Verification items for the finished model (mm, model axes). A direction names the side the tool comes from. Give positions to 0.01 mm unless a question says otherwise; leave off trailing zeros. Order: outer loops, then holes, each group sorted by start corner. A loop starts at its lowest first (then second) coordinate and runs counter-clockwise, first axis right, second up. Notation, with made-up numbers: (52, 66) -> (88, 66) arc R31 cw to (88, 93) -> close; hole circle Ø3 at (35, 33). An arc over 180 degrees is marked (long way). Return JSON: item names as keys, results as strings. Group by question number.
(1) Thickness scan on line 1 along X through (y, z) = (9.5, -14); line 2 along X through (y, z) = (2, -7); line 3 along Y through (x, z) = (20.5, 17.5). Record the ranges inside material, lowest first.
(2) Cross-section at D-D on x = 0. Enter the section's corners in (y, z), then the cut area to 3 significant figures.
(3) Tool access check on faces 4 (the face through (-22.43, 1.48, 23.27)), 5 (the face through (-28, 5, 5)), 6 (the face through (26, 5, -10)), 7 (the face through (24, 7, -10)). Record the directions out of +Z, -Z, +X, -X, +Y, -Y that give a thin tool (end or side, any length) a straight path to the whole face; none if there is none.
(4) Cross-section at C-C on z = -23. Enter the section's corners in (x, y).
(5) Release check for a two-part mould opening along X. For faces 1 (the face through (20, 1, 24.662)), 2 (the face through (-26, 5, -27)), 3 (the face through (28, 5, 5)) record: pulls with the +X half, pulls with the -X half, needs draft (parallel to the pull), parting line crosses it, or undercut.
(6) Depth check by flat-ended pin: pin 1 Ø5 at (x, y) = (-17, 4.5) entering from -Z; pin 2 Ø1.6 at (x, y) = (24.5, 7) entering from +Z; pin 3 Ø1 at (y, z) = (6.5, -8) entering from -X; pin 4 Ø4.5 at (x, z) = (0, 14) entering from -Y. Enter the tip coordinate at first touch or a pass-through.
(7) Cross-section at A-A on y = 6. Enter the section's corners in (x, z).
(8) Cross-section at B-B on x = -8. Enter the section's corners in (y, z).
from build123d import *

# Parameters (mm, degrees)
SKETCH1_W               = 52
SKETCH1_H               = 60
BOSS_EXTRUDE1_DEPTH     = 10
CUT_EXTRUDE1_DEPTH      = 5
SKETCH3_R               = 1.25
CUT_EXTRUDE2_DEPTH      = 5
CUT_EXTRUDE3_DEPTH      = 3
SKETCH6_W               = 24
SKETCH6_H               = 30
CUT_EXTRUDE4_DEPTH      = 41.938978981
SKETCH7_W               = 3
SKETCH7_H               = 10
BOSS_EXTRUDE2_DEPTH     = 10
LPATTERN1_COUNT         = 2
LPATTERN1_PITCH         = 20
MIRROR1_COPY_1_SKETCH_W = 3
MIRROR1_COPY_1_SKETCH_H = 10
MIRROR1_COPY_1_DEPTH    = 10
SKETCH8_W               = 48
SKETCH8_H               = 40
CUT_EXTRUDE5_DEPTH      = 2


with BuildPart() as part:
    # Sketch1 → Boss-Extrude1 (new body)
    with BuildSketch(Plane(origin=(0, 0, 0), x_dir=(1, 0, 0), z_dir=(0, 1, 0))):
        Rectangle(SKETCH1_W, SKETCH1_H)
    extrude(amount=BOSS_EXTRUDE1_DEPTH)

    # Sketch2 → Cut-Extrude1 (cut)
    with BuildSketch(Plane(origin=(0, 10, 0), x_dir=(1, 0, 0), z_dir=(0, 1, 0))):
        Polygon((-26, -30), (26, -30), (26, -10), (24, -10), (24, 30), (-24, 30), (-24, -10), (-26, -10), align=None)
    extrude(amount=-CUT_EXTRUDE1_DEPTH, mode=Mode.SUBTRACT)

    # Sketch3 → Cut-Extrude2 (cut)
    with BuildSketch(Plane(origin=(0, 5, 0), x_dir=(1, 0, 0), z_dir=(0, 1, 0))):
        with Locations(Location((-20, -21.847557332, 0), (0, 0, 270))):
            Circle(SKETCH3_R)
        with Locations(Location((0, -13.847557332, 0), (0, 0, 270))):
            Circle(SKETCH3_R)
        with Locations(Location((20, -21.847557332, 0), (0, 0, 270))):
            Circle(SKETCH3_R)
    extrude(amount=-CUT_EXTRUDE2_DEPTH, mode=Mode.SUBTRACT)

    # Sketch5 → Cut-Extrude3 (cut)
    with BuildSketch(Plane.XZ):
        Polygon((-18.375, 24.662139894), (-21.625, 24.662139894), (-23.25, 21.847557332), (-21.625, 19.03297477), (-18.375, 19.03297477), (-16.75, 21.847557332), align=None)
        Polygon((1.625, 16.662139894), (-1.625, 16.662139894), (-3.25, 13.847557332), (-1.625, 11.03297477), (1.625, 11.03297477), (3.25, 13.847557332), align=None)
        Polygon((21.625, 24.662139894), (18.375, 24.662139894), (16.75, 21.847557332), (18.375, 19.03297477), (21.625, 19.03297477), (23.25, 21.847557332), align=None)
    extrude(amount=-CUT_EXTRUDE3_DEPTH, mode=Mode.SUBTRACT)

    # Sketch6 → Cut-Extrude4 (cut, through all)
    with BuildSketch(Plane.XZ):
        with Locations((0, -5)):
            Rectangle(SKETCH6_W, SKETCH6_H)
    extrude(amount=-CUT_EXTRUDE4_DEPTH, mode=Mode.SUBTRACT)

    # Sketch7 → Boss-Extrude2 (add)
    with BuildSketch(Plane(origin=(0, 10, 0), x_dir=(1, 0, 0), z_dir=(0, 1, 0))):
        with Locations((-27.5, 20)):
            Rectangle(SKETCH7_W, SKETCH7_H)
    boss_extrude2 = extrude(amount=-BOSS_EXTRUDE2_DEPTH)

    # LPattern1: Boss-Extrude2 ×2
    with Locations(*[(0, 0, i * LPATTERN1_PITCH) for i in range(1, LPATTERN1_COUNT)]):
        add(boss_extrude2)

    # Mirror1: Boss-Extrude2 across plane
    add(boss_extrude2.mirror(Plane(origin=(0, 0, 0), x_dir=(0, 0, 1), z_dir=(1, 0, 0))))

    # Mirror1 copy 1 sketch → Mirror1 copy 1 (add)
    with BuildSketch(Plane(origin=(0, 10, 20), x_dir=(-1, 0, 0), z_dir=(0, 1, 0))):
        with Locations((-27.5, -20)):
            Rectangle(MIRROR1_COPY_1_SKETCH_W, MIRROR1_COPY_1_SKETCH_H)
    extrude(amount=-MIRROR1_COPY_1_DEPTH)

    # Sketch8 → Cut-Extrude5 (cut)
    with BuildSketch(Plane(origin=(0, 5, 0), x_dir=(1, 0, 0), z_dir=(0, 1, 0))):
        with Locations((0, 10)):
            Rectangle(SKETCH8_W, SKETCH8_H)
    extrude(amount=-CUT_EXTRUDE5_DEPTH, mode=Mode.SUBTRACT)


solid = part.part
Verdict:
{
 "1": {"line 1": "-26 to -24, 24 to 26", "line 2": "-26 to -12, 12 to 26", "line 3": "0 to 5"},
 "2": {"outline": "(0, -30) -> (3, -30) -> (3, -20) -> (0, -20) -> close; (0, 10) -> (5, 10) -> (5, 12.6) -> (3, 12.6) -> (3, 11.03) -> (0, 11.03) -> close; (0, 16.66) -> (3, 16.66) -> (3, 15.1) -> (5, 15.1) -> (5, 30) -> (0, 30) -> close", "area": "108 mm²"},
 "3": {"face 4": "-Y", "face 5": "+Z, -X, +Y, -Y", "face 6": "+X, +Y, -Y", "face 7": "-Z, +Y"},
 "4": {"outline": "(-29, 0) -> (29, 0) -> (29, 10) -> (24, 10) -> (24, 3) -> (-24, 3) -> (-24, 10) -> (-29, 10) -> close"},
 "5": {"face 1": "undercut", "face 2": "pulls with the -X half", "face 3": "needs draft"},
 "6": {"pin 1": "z = -30", "pin 2": "z = 10", "pin 3": "x = -26", "pin 4": "y = 3"},
 "7": {"outline": "(-29, -25) -> (-26, -25) -> (-26, -30) -> (-24, -30) -> (-24, 10) -> (-26, 10) -> (-26, 5) -> (-29, 5) -> (-29, -5) -> (-26, -5) -> (-26, -15) -> (-29, -15) -> close; (24, -30) -> (26, -30) -> (26, -25) -> (29, -25) -> (29, -15) -> (26, -15) -> (26, -5) -> (29, -5) -> (29, 5) -> (26, 5) -> (26, 10) -> (24, 10) -> close"},
 "8": {"outline": "(0, -30) -> (3, -30) -> (3, -20) -> (0, -20) -> close; (0, 10) -> (5, 10) -> (5, 30) -> (0, 30) -> close"}
}
